Geometry: final body of the model. Coordinates: model frame, mm. Face numbers are marked on the shaded views. Coordinates: 2 decimals unless noted, no trailing zeros. Loops run counter-clockwise (first coordinate to the right, second up) from the corner with the lowest first, then second, coordinate; pieces in that order, holes last. Notation, with made-up numbers: (-23, -22.5) - (-11, -22.5) arc R26 cw to (-11, 6.5) - close; hole circle Ø6 at (28.25, 14). An arc over 180 degrees is marked (long way). Answer in a Markdown table with one row per item.
from build123d import *

# Parameters (mm, degrees)
BOSS_EXTRUDE1_DEPTH     = 2.54
SKETCH4_R               = 1.905
SKETCH4_W               = 20.32
SKETCH4_H               = 50.8
CUT_EXTRUDE2_DEPTH      = 25.4
SKETCH5_W               = 20.32
SKETCH5_H               = 7.493
CUT_EXTRUDE3_DEPTH      = 5.08
SKETCH8_W               = 12.7
SKETCH8_H               = 2.54
SKETCH8_W_2             = 2.54
SKETCH8_H_2             = 12.7
CUT_EXTRUDE5_DEPTH      = 5.08
BOSS_EXTRUDE2_DEPTH     = 5.842
SKETCH10_R              = 1.27
CUT_EXTRUDE6_DEPTH      = 1
CUT_EXTRUDE6_DEPTH_BACK = 9.382
SKETCH6_R               = 1.27
CUT_EXTRUDE7_DEPTH      = 1
CUT_EXTRUDE7_DEPTH_BACK = 9.382


with BuildPart() as part:
    # Sketch1 → Boss-Extrude1 (new body)
    with BuildSketch(Plane.XY):
        with BuildLine():
            Line((-3.314058103, 6.35), (48.26, 6.35))
            ThreePointArc((48.26, 6.35), (51.852102448, 4.862102448), (53.34, 1.27))
            Line((53.34, 1.27), (53.34, -92.71))
            ThreePointArc((53.34, -92.71), (51.852102448, -96.302102448), (48.26, -97.79))
            Line((48.26, -97.79), (16.846989059, -97.79))
            ThreePointArc((16.846989059, -97.79), (15.638688158, -97.644208035), (14.499741809, -97.215200367))
            Line((14.499741809, -97.215200367), (-16.7505185, -80.933552139))
            ThreePointArc((-16.7505185, -80.933552139), (-18.059258376, -79.955412607), (-18.989802686, -78.61241436))
            Line((-18.989802686, -78.61241436), (-28.309569459, -59.040904135))
            ThreePointArc((-28.309569459, -59.040904135), (-28.795802898, -57.127870198), (-28.51617555, -55.173917704))
            Line((-28.51617555, -55.173917704), (-8.107195629, 2.952923842))
            ThreePointArc((-8.107195629, 2.952923842), (-6.251501454, 5.414614163), (-3.314058103, 6.35))
        make_face()
    extrude(amount=BOSS_EXTRUDE1_DEPTH)

    # Sketch4 → Cut-Extrude2 (cut)
    with BuildSketch(Plane(origin=(0, 0, 0), x_dir=(-1, 0, 0), z_dir=(0, 0, -1))):
        with Locations((-39.37, -17.78)):
            Circle(SKETCH4_R)
        with Locations((-34.29, -17.78)):
            Circle(SKETCH4_R)
        with Locations((-39.37, -27.94)):
            Circle(SKETCH4_R)
        with Locations((-34.29, -27.94)):
            Circle(SKETCH4_R)
        with Locations((-41.91, -45.72)):
            Circle(SKETCH4_R)
        with Locations((-36.83, -45.72)):
            Circle(SKETCH4_R)
        with Locations((-44.45, -64.77)):
            Circle(SKETCH4_R)
        with Locations((-39.37, -64.77)):
            Circle(SKETCH4_R)
        with Locations((-44.45, -83.82)):
            Circle(SKETCH4_R)
        with Locations((-39.37, -83.82)):
            Circle(SKETCH4_R)
        with Locations((-24.257, -17.78)):
            Circle(SKETCH4_R)
        with Locations((-19.939, -17.78)):
            Circle(SKETCH4_R)
        with Locations((-24.257, -27.94)):
            Circle(SKETCH4_R)
        with Locations((-19.939, -27.94)):
            Circle(SKETCH4_R)
        with Locations((-26.162, -45.72)):
            Circle(SKETCH4_R)
        with Locations((-21.082, -45.72)):
            Circle(SKETCH4_R)
        with Locations((-27.686, -64.77)):
            Circle(SKETCH4_R)
        with Locations((-22.606, -64.77)):
            Circle(SKETCH4_R)
        with Locations((-7.62, -26.543)):
            Rectangle(SKETCH4_W, SKETCH4_H)
    extrude(amount=-CUT_EXTRUDE2_DEPTH, mode=Mode.SUBTRACT)

    # Sketch5 → Cut-Extrude3 (cut)
    with BuildSketch(Plane.XY.offset(2.54)):
        with Locations((7.62, 2.6035)):
            Rectangle(SKETCH5_W, SKETCH5_H)
    extrude(amount=-CUT_EXTRUDE3_DEPTH, mode=Mode.SUBTRACT)

    # Sketch8 → Cut-Extrude5 (cut)
    with BuildSketch(Plane.XY.offset(2.54)):
        with Locations((29.972, -84.5566)):
            Rectangle(SKETCH8_W, SKETCH8_H)
        with Locations((20.066, -78.359)):
            Rectangle(SKETCH8_W_2, SKETCH8_H_2)
        with Locations((13.208, -81.026)):
            Rectangle(SKETCH8_W_2, SKETCH8_H_2)
        with Locations((5.588, -78.486)):
            Rectangle(SKETCH8_W_2, SKETCH8_H_2)
    extrude(amount=-CUT_EXTRUDE5_DEPTH, mode=Mode.SUBTRACT)

    # Sketch9 → Boss-Extrude2 (add)
    with BuildSketch(Plane(origin=(0, 0, 0), x_dir=(-1, 0, 0), z_dir=(0, 0, -1))):
        with BuildLine():
            Line((-48.26, -97.79), (-48.26, 1.27))
            Line((-48.26, 1.27), (-17.78, 1.27))
            Line((-17.78, 1.27), (-17.78, 6.35))
            Line((-17.78, 6.35), (-48.26, 6.35))
            ThreePointArc((-48.26, 6.35), (-51.852102448, 4.862102448), (-53.34, 1.27))
            Line((-53.34, 1.27), (-53.34, -92.71))
            ThreePointArc((-53.34, -92.71), (-51.852102448, -96.302102448), (-48.26, -97.79))
        make_face()
        with BuildLine():
            Line((2.54, 0.820424909), (2.54, -82.609215784))
            Line((2.54, -82.609215784), (-16.846989059, -92.71))
            Line((-16.846989059, -92.71), (-16.846989059, -97.79))
            ThreePointArc((-16.846989059, -97.79), (-15.638688158, -97.644208035), (-14.499741809, -97.215200367))
            Line((-14.499741809, -97.215200367), (16.7505185, -80.933552139))
            ThreePointArc((16.7505185, -80.933552139), (18.059258376, -79.955412607), (18.989802686, -78.61241436))
            Line((18.989802686, -78.61241436), (28.309569459, -59.040904135))
            ThreePointArc((28.309569459, -59.040904135), (28.795802898, -57.127870198), (28.51617555, -55.173917704))
            Line((28.51617555, -55.173917704), (8.107195629, 2.952923842))
            ThreePointArc((8.107195629, 2.952923842), (6.251501454, 5.414614163), (3.314058103, 6.35))
            Line((3.314058103, 6.35), (2.54, 6.35))
            Line((2.54, 6.35), (2.54, 0.820424909))
        make_face()
    extrude(amount=BOSS_EXTRUDE2_DEPTH)

    # Sketch10 → Cut-Extrude6 (cut, two sides)
    with BuildSketch(Plane.XY.offset(2.54)) as cut_extrude6_sk:
        with Locations((48.0822, 2.286)):
            Circle(SKETCH10_R)
        with Locations((-3.718687848, 1.651)):
            Circle(SKETCH10_R)
        with Locations((-25.012261453, -59.761967182)):
            Circle(SKETCH10_R)
    extrude(amount=CUT_EXTRUDE6_DEPTH, mode=Mode.SUBTRACT)
    extrude(cut_extrude6_sk.sketch, amount=-CUT_EXTRUDE6_DEPTH_BACK, mode=Mode.SUBTRACT)

    # Sketch6 → Cut-Extrude7 (cut, two sides)
    with BuildSketch(Plane.XY.offset(2.54)) as cut_extrude7_sk:
        with Locations((1.6002, -2.4384)):
            Circle(SKETCH6_R)
        with Locations((44.2976, -2.4384)):
            Circle(SKETCH6_R)
        with Locations((-17.4498, -57.15)):
            Circle(SKETCH6_R)
        with Locations((-10.5918, -71.3486)):
            Circle(SKETCH6_R)
        with Locations((18.796, -86.5378)):
            Circle(SKETCH6_R)
    extrude(amount=CUT_EXTRUDE7_DEPTH, mode=Mode.SUBTRACT)
    extrude(cut_extrude7_sk.sketch, amount=-CUT_EXTRUDE7_DEPTH_BACK, mode=Mode.SUBTRACT)


solid = part.part
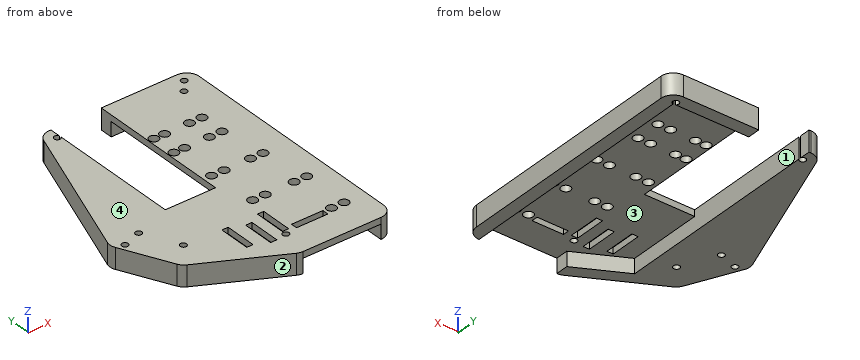
(1) First-contact query: pin 1 Ø5 at (x, y) = (30, -65) entering from -Z; pin 2 Ø4.5 at (x, z) = (36, -4) entering from -Y; pin 3 Ø3 at (y, z) = (-8, -4.5) entering from -X. Flat tips, straight axial feed; report the tip coordinate or a pass-through.
Verdict:
| item | result |
|---|---|
| pin 1 | stops at z = 0 |
| pin 2 | stops at y = 1.27 |
| pin 3 | stops at x = -12.48 |
(2) Cut plane C-C on y = -64.77. Output: boundary loops of the cut face in (x, z) (3 decimals), then the cut area to 3 significant figures.
Verdict:
| item | result |
|---|---|
| outline | (-25.581, -5.842) - (-2.54, -5.842) - (-2.54, 0) - (20.701, 0) - (20.701, 2.54) - (-25.581, 2.54) - close; (24.511, 0) - (25.781, 0) - (25.781, 2.54) - (24.511, 2.54) - close; (29.591, 0) - (37.465, 0) - (37.465, 2.54) - (29.591, 2.54) - close; (41.275, 0) - (42.545, 0) - (42.545, 2.54) - (41.275, 2.54) - close; (46.355, 0) - (48.26, 0) - (48.26, -5.842) - (53.34, -5.842) - (53.34, 2.54) - (46.355, 2.54) - close |
| area | 326 mm² |
(3) Pull-direction query (X, two-part tool) for the marked faces 1, 2, 3 and 4; classes: pulls with the +X half, pulls with the -X half, needs draft (parallel to the pull), parting line crosses it, or undercut.
Verdict:
| item | result |
|---|---|
| face 1 | undercut |
| face 2 | pulls with the -X half |
| face 3 | undercut |
| face 4 | needs draft |
(4) Ray query, probe 1 along Y at (x, z) = (44.45, 1.3) (3 decimals); probe 2 along Z at (x, y) = (12, -55); probe 3 along Y at (x, z) = (25.5, -1.25). Return the intervals inside material, ascending.
Verdict:
| item | result |
|---|---|
| probe 1 | y = -97.79 to -85.725, -81.915 to -66.675, -62.865 to -3.699, -1.178 to 6.35 |
| probe 2 | z = 0 to 2.54 |
| probe 3 | y = 1.27 to 6.35 |
(5) Cut plane B-B on y = -17.78. Output: boundary loops of the cut face in (x, z) (3 decimals).
Verdict:
| item | result |
|---|---|
| outline | (-15.387, -5.842) - (-2.54, -5.842) - (-2.54, 2.54) - (-15.387, 2.54) - close; (17.78, 0) - (18.034, 0) - (18.034, 2.54) - (17.78, 2.54) - close; (21.844, 0) - (22.352, 0) - (22.352, 2.54) - (21.844, 2.54) - close; (26.162, 0) - (32.385, 0) - (32.385, 2.54) - (26.162, 2.54) - close; (36.195, 0) - (37.465, 0) - (37.465, 2.54) - (36.195, 2.54) - close; (41.275, 0) - (48.26, 0) - (48.26, -5.842) - (53.34, -5.842) - (53.34, 2.54) - (41.275, 2.54) - close |
(6) Cut plane D-D on y = -36. Output: boundary loops of the cut face in (x, z), then the cut area to 3 significant figures.
Verdict:
| item | result |
|---|---|
| outline | (-21.78, -5.84) - (-2.54, -5.84) - (-2.54, 2.54) - (-21.78, 2.54) - close; (17.78, 0) - (48.26, 0) - (48.26, -5.84) - (53.34, -5.84) - (53.34, 2.54) - (17.78, 2.54) - close |
| area | 281 mm² |
(7) Cut plane A-A on z = -4. Output: boundary loops of the cut face in (x, y).
Verdict:
| item | result |
|---|---|
| outline | (-28.52, -55.17) arc R5.08 ccw to (-28.31, -59.04) - (-18.99, -78.61) arc R5.08 ccw to (-16.75, -80.93) - (14.5, -97.22) arc R5.08 ccw to (16.85, -97.79) - (16.85, -92.71) - (-2.54, -82.61) - (-2.54, 1.18) arc R1.27 cw (long way) to (-2.54, 2.12) - (-2.54, 6.35) - (-3.31, 6.35) arc R5.08 ccw to (-8.11, 2.95) - close; (17.78, 1.27) - (47.32, 1.27) arc R1.27 cw (long way) to (48.26, 1.03) - (48.26, -97.79) arc R5.08 ccw to (53.34, -92.71) - (53.34, 1.27) arc R5.08 ccw to (48.26, 6.35) - (17.78, 6.35) - close; hole circle Ø2.54 at (-25.01, -59.76); hole circle Ø2.54 at (-17.45, -57.15); hole circle Ø2.54 at (-10.59, -71.35) |
